from build123d import *

# Parameters (mm, degrees)
SKETCH1_R              = 4
SKETCH1_R_2            = 2.5
BOSS_EXTRUDE1_DEPTH    = 11
M3_TAPPED_HOLE1_REACH  = 16.177
M3_TAPPED_HOLE1_BORE_R = 1.25
SKETCH8_R              = 3.5


with BuildPart() as part:
    # Sketch1 → Boss-Extrude1 (new body)
    with BuildSketch(Plane(origin=(0, 0, 0), x_dir=(1, 0, 0), z_dir=(0, 1, 0))):
        with Locations(Location((0, 0, 0), (0, 0, 270))):
            Circle(SKETCH1_R)
        with Locations(Location((0, 0, 0), (0, 0, 270))):
            Circle(SKETCH1_R_2, mode=Mode.SUBTRACT)
    extrude(amount=BOSS_EXTRUDE1_DEPTH)

    # M3 Tapped Hole1 bore → M3 Tapped Hole1 (cut, up to next)
    with BuildSketch(Plane.XY.offset(4), mode=Mode.PRIVATE) as m3_tapped_hole1_sk1:
        with Locations((0, 8.5)):
            Circle(M3_TAPPED_HOLE1_BORE_R)
    m3_tapped_hole1_tool1 = extrude(m3_tapped_hole1_sk1.sketch, amount=-M3_TAPPED_HOLE1_REACH, mode=Mode.PRIVATE) & part.part
    add(m3_tapped_hole1_tool1.solids().sort_by_distance((0, 8.5, 4))[0], mode=Mode.SUBTRACT)

    # Sketch8 → Cut-Revolve2 (revolve, cut)
    with BuildSketch(Plane.XY, mode=Mode.PRIVATE) as cut_revolve2_sk:
        with Locations((6.75, 3.5)):
            Circle(SKETCH8_R)
    revolve(cut_revolve2_sk.sketch.rotate(Axis((0, 11, 0), (0, -1, 0)), 90), axis=Axis((0, 11, 0), (0, -1, 0)), mode=Mode.SUBTRACT)


solid = part.part
Model file for the job. Use its own axes, mm. Coordinates: 2 decimals unless noted, no trailing zeros. Write each loop counter-clockwise with the first axis right and the second up, starting at its lowest first coordinate (ties: lowest second). Pieces come first, ordered by that corner, then holes. Notation, with made-up numbers: (28, 11.25) - (68, 11.25) arc R25 cw to (68, 46.25) - close; hole circle Ø9 at (7, 36). An arc over 180 degrees is marked (long way). Write each question's results on one line, items separated by ' | '. Start each with the question number.
1) Cut at D-D (y = 8.5). Write the cut outline in (x, z), then the cut area to 3 significant figures.
2) Probe line 1 along Y through (x, z) = (0, 3.15); line 2 along X through (y, z) = (6.75, 0); line 3 along X through (y, z) = (2.25, 1.5). List the from-to ranges inside material, lowest first. Write a range as from..to.
3) Cut at B-B (z = 0). Write the cut outline in (x, y).
4) Cut at A-A (x = 0). Write the cut outline in (y, z), then the cut area to 3 significant figures.
5) Flat gauge pins, fed straight in: P1, Ø4, axis at x = 2, z = 0, coming from the -Y side; P2, Ø4, axis at x = 0, z = 0, coming from the -Y side; P3, Ø1.5, axis at y = 3, z = 2, coming from the +X side. Where does each tip first touch, or does it go through?
6) Cut at C-C (y = 10). Write the cut outline in (x, z).
7) Mould opens along Y. For faces 1 (the face through (1.155, 8.021, 3.095)), 2 (the face through (-3.905, 0.658, -0.867)), 3 (the face through (2, 0, 2)) say: pulls with the +Y half, pulls with the -Y half, needs draft (parallel to the pull), parting line crosses it, or undercut.
Returned:
1) outline: (-1.25, 2.17) - (-1.25, 3.8) arc R4 ccw (long way) to (1.25, 3.8) - (1.25, 2.17) arc R2.5 cw (long way) to start | area: 26.8 mm^2
2) line 1: 0..7.25, 9.75..11 | line 2: -4..-2.5, 2.5..4 | line 3: -3.14..-2, 2..3.14
3) outline: (-4, 0) - (-2.5, 0) - (-2.5, 11) - (-4, 11) - (-4, 5.67) arc R3.5 cw to (-4, 1.33) - close; (2.5, 0) - (4, 0) - (4, 1.33) arc R3.5 cw to (4, 5.67) - (4, 11) - (2.5, 11) - close
4) outline: (0, -4) - (1.33, -4) arc R3.5 cw to (5.67, -4) - (11, -4) - (11, -2.5) - (0, -2.5) - close; (0, 2.5) - (7.25, 2.5) - (7.25, 4) - (5.67, 4) arc R3.5 cw to (1.33, 4) - (0, 4) - close; (9.75, 2.5) - (11, 2.5) - (11, 4) - (9.75, 4) - close | area: 24.8 mm^2
5) P1: y = 0 | P2: through | P3: x = 3.08
6) outline: circle Ø8 at (0, 0); hole circle Ø5 at (0, 0)
7) face 1: undercut | face 2: needs draft | face 3: pulls with the -Y half
